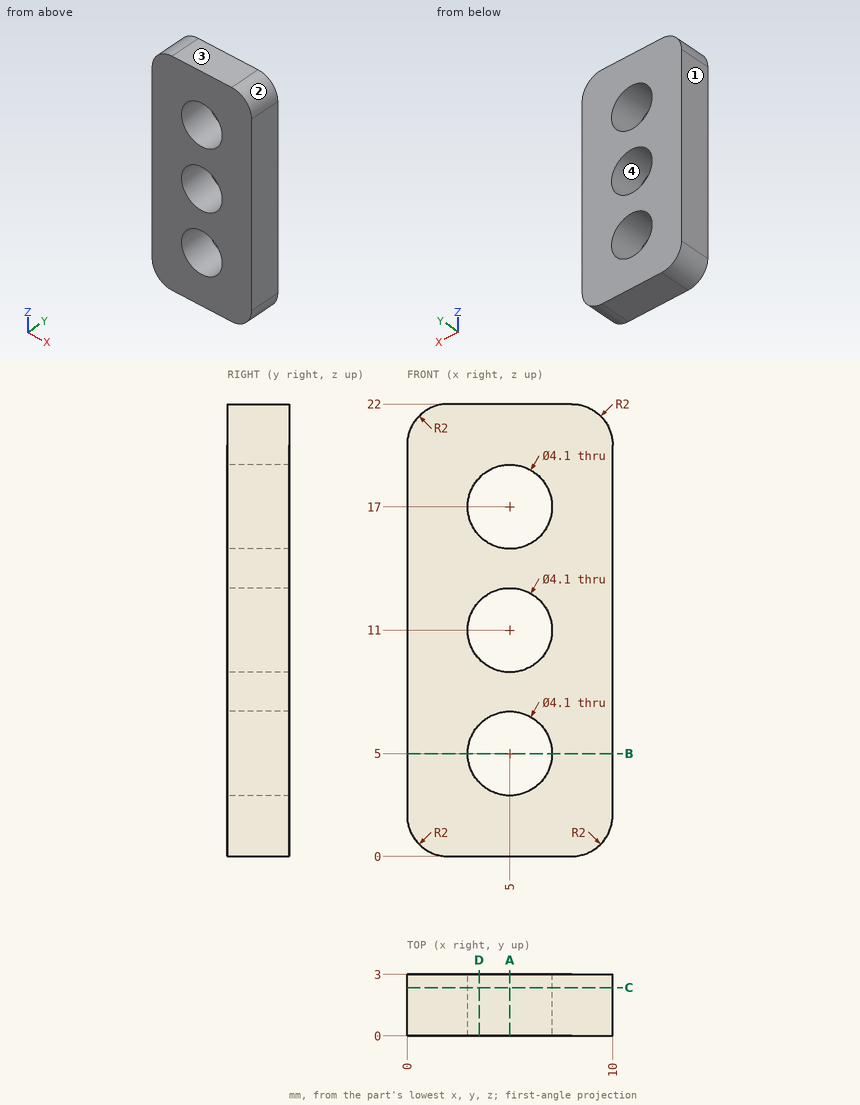
Job drawing, mm, ordinate dimensions from the low corner. One solid piece. Coordinates: 2 decimals unless noted, no trailing zeros. Write each loop counter-clockwise with the first axis right and the second up, starting at its lowest first coordinate (ties: lowest second). Pieces come first, ordered by that corner, then holes.
Item 1: Probe line 1 (Z direction, x = 5, y = 2.4); line 2 (Z direction, x = 6.25, y = 2.25); line 3 (X direction, y = 1.4, z = 10.5). List the from-to ranges inside material, lowest first.
Item 2: Slice it at C-C (y = 2.35). Write the cut outline in (x, z).
Item 3: Slice it at A-A (x = 5). Write the cut outline in (y, z), and give its area (3 significant figures).
Item 4: Slice it at D-D (x = 3.5). Write the cut outline in (y, z), and give its area (3 significant figures).
Item 5: Pin check, flat tip, straight feed: pin 1 (3.5 mm diameter, centred on x = 5, z = 17, fed in from +Y). Stop position of the tip, or through.
Item 6: Slice it at B-B (z = 5). Write the cut outline in (x, y), and give its area (3 significant figures).
Item 7: Mould opens along X. For the marked faces 1, 2, 3 and 4 say: released by +X, released by -X, zero draft, split by the parting line, or undercut.
Results found:
1. line 1: z = 0 to 2.95, 7.05 to 8.95, 13.05 to 14.95, 19.05 to 22
1. line 2: z = 0 to 3.38, 6.62 to 9.38, 12.62 to 15.38, 18.62 to 22
1. line 3: x = 0 to 3.01, 6.99 to 10
2. outline: (0, 2) arc R2 ccw to (2, 0) - (8, 0) arc R2 ccw to (10, 2) - (10, 20) arc R2 ccw to (8, 22) - (2, 22) arc R2 ccw to (0, 20) - close; hole circle Ø4.1 at (5, 5); hole circle Ø4.1 at (5, 11); hole circle Ø4.1 at (5, 17)
3. outline: (0, 0) - (3, 0) - (3, 2.95) - (0, 2.95) - close; (0, 7.05) - (3, 7.05) - (3, 8.95) - (0, 8.95) - close; (0, 13.05) - (3, 13.05) - (3, 14.95) - (0, 14.95) - close; (0, 19.05) - (3, 19.05) - (3, 22) - (0, 22) - close
3. area: 29.1 mm2
4. outline: (0, 0) - (3, 0) - (3, 3.6) - (0, 3.6) - close; (0, 6.4) - (3, 6.4) - (3, 9.6) - (0, 9.6) - close; (0, 12.4) - (3, 12.4) - (3, 15.6) - (0, 15.6) - close; (0, 18.4) - (3, 18.4) - (3, 22) - (0, 22) - close
4. area: 40.8 mm2
5. pin 1: passes through
6. outline: (0, 0) - (2.95, 0) - (2.95, 3) - (0, 3) - close; (7.05, 0) - (10, 0) - (10, 3) - (7.05, 3) - close
6. area: 17.7 mm2
7. face 1: released by -X
7. face 2: released by +X
7. face 3: zero draft
7. face 4: undercut
